from build123d import *

# Parameters (mm, degrees)
F0_R      = 2.5146
F1_DEPTH  = 10.16
F2_R      = 1.2446
F3_DEPTH  = 17.78
F3_FACE_R = 1.2446
F5_R      = 0.422561
F7_R      = 1.27
F8_DEPTH  = 25.4
F9_DEPTH  = 25.4
F11_DEPTH = 1.2192
F12_DEPTH = 1.2192


with BuildPart() as f1:
    # F0 (on Front) → F1 (new body)
    with BuildSketch(Plane.XZ):
        Circle(F0_R)
    extrude(amount=F1_DEPTH)

    # F2 (on face) → F3 (join)
    with BuildSketch(Plane.XZ.offset(10.16)):
        Circle(F2_R)
    extrude(amount=F3_DEPTH)

    # F3_face (on face) → F6 section 0
    with BuildSketch(Plane.XZ.offset(27.94)):
        Circle(F3_FACE_R)
    # F5 (on offset) → F6 section 1
    with BuildSketch(Plane.XZ.offset(30.48)):
        Circle(F5_R)
    loft()

    # F7 (on Right) → F8 (cut)
    with BuildSketch(Plane.YZ):
        with Locations((-6.35, 0)):
            Circle(F7_R)
    extrude(amount=-F8_DEPTH, mode=Mode.SUBTRACT)

    # F7 (on Right) → F9 (cut)
    with BuildSketch(Plane.YZ):
        with Locations((-6.35, 0)):
            Circle(F7_R)
    extrude(amount=F9_DEPTH, mode=Mode.SUBTRACT)

    # F10 (on Right) → F11 (join)
    with BuildSketch(Plane.YZ):
        Polygon((0, -2.54), (0, 0), (-5.08, 0), (-5.08, -2.54), (-5.08, -5.08), align=None)
    extrude(amount=F11_DEPTH)

    # F10 (on Right) → F12 (join)
    with BuildSketch(Plane.YZ):
        Polygon((0, -2.54), (0, 0), (-5.08, 0), (-5.08, -2.54), (-5.08, -5.08), align=None)
    extrude(amount=-F12_DEPTH)


solid = f1.part
Geometry check sheet. Reference: the model listing, model coordinates, mm. A direction names the side the tool comes from. Round coordinates to 2 decimals unless told otherwise and drop trailing zeros. Loops run counter-clockwise (first coordinate to the right, second up) from the corner with the lowest first, then second, coordinate; pieces in that order, holes last. Notation, with made-up numbers: (-1.5, -6) - (33.5, -6) arc R11 cw to (33.5, 8) - close; hole circle Ø4 at (-5.75, -15). An arc over 180 degrees is marked (long way). Answer as CSV lines item,"result".
(1) Release check for a two-part mould opening along Z. For faces 4 (the face through (-0.584, -29.51, -0.448)), 5 (the face through (1.219, -3, -3)), 6 (the face through (0.02, -2.58, -3.83)) record: released by +Z, released by -Z, zero draft, split by the parting line, or undercut.
Output values:
face 4,"split by the parting line"
face 5,"zero draft"
face 6,"released by -Z"
(2) Cross-section at B-B, the plane y = -6.35. Enter the section's corners in (x, z).
Output values:
outline,"(-2.17, -1.27) arc R2.51 ccw to (2.17, -1.27) - close; (-2.17, 1.27) - (2.17, 1.27) arc R2.51 ccw to start"
(3) Set-up check for faces 1 (the face through (-0.327, -5.009, 2.493)), 2 (the face through (0, -30.48, 0)), 3 (the face through (-1.219, -3, -3)): record each of +Z, -Z, +X, -X, +Y, -Y from which the full face is reachable in a straight line by a thin tool's end or side.
Output values:
face 1,"-Y"
face 2,"+Z, -Z, +X, -X, -Y"
face 3,"-Z, -X, +Y, -Y"
(4) Material ranges on line 1 along Y through (x, z) = (1.3, 0); line 2 along Z through (x, y) = (-0.6, -6.35); line 3 along X through (y, z) = (-3, -2.25), recorded low to high.
Output values:
line 1,"y = -10.16 to -7.62, -5.08 to 0"
line 2,"z = -2.44 to -1.27, 1.27 to 2.44"
line 3,"x = -1.22 to 1.22"
(5) Cross-section at A-A, the plane x = -1.7. Enter the section's corners in (y, z).
Output values:
outline,"(-10.16, -1.85) - (0, -1.85) - (0, 1.85) - (-10.16, 1.85) - close; hole circle Ø2.54 at (-6.35, 0)"
(6) Cross-section at C-C, the plane z = -4. Enter the section's corners in (x, y), and give its area (3 significant figures).
Output values:
outline,"(-1.22, -5.08) - (1.22, -5.08) - (1.22, -2.92) - (-1.22, -2.92) - close"
area,"5.27 mm²"
(7) Cross-section at D-D, the plane y = -22. Enter the section's corners in (x, z).
Output values:
outline,"circle Ø2.49 at (0, 0)"
(8) Depth check by flat-ended pin: pin 1 Ø1.5 at (y, z) = (-6.35, 0) entering from +X; pin 2 Ø3 at (y, z) = (-3, -3.5) entering from +X; pin 3 Ø2 at (x, y) = (2, -25.5) entering from -Z; pin 4 Ø2.5 at (y, z) = (-1.5, -3.5) entering from -X. Enter the tip coordinate at first touch or a pass-through.
Output values:
pin 1,"passes through"
pin 2,"stops at x = 1.52"
pin 3,"stops at z = -0.74"
pin 4,"stops at x = -1.22"
